```python
from build123d import *

# Parameters (mm, degrees)
F2_R      = 2
F3_DEPTH  = 20
F4_R      = 4
F5_DEPTH  = 20
F8_DEPTH  = 1.4
F9_R      = 3
F10_DEPTH = 8
F9_R_2    = 5
F11_DEPTH = 0.4


with BuildPart() as f1:
    # F0 (on Front) → F1 (revolve)
    with BuildSketch(Plane.XZ):
        Polygon((0, 15), (0, 0), (48, 0), (48, 4.5), (36, 4.5), (36, 7), (3, 7), (3, 11), (2.8, 11), (2.8, 15), align=None)
    revolve(axis=Axis((24, 0, 0), (-1, 0, 0)))

    # F2 (on face) → F3 (cut)
    with BuildSketch(Plane.YZ.offset(48)):
        Circle(F2_R)
    extrude(amount=-F3_DEPTH, mode=Mode.SUBTRACT)

    # F4 (on face) → F5 (cut)
    with BuildSketch(Plane(origin=(0, 0, 0), x_dir=(0, -1, 0), z_dir=(-1, 0, 0))):
        Circle(F4_R)
    extrude(amount=-F5_DEPTH, mode=Mode.SUBTRACT)

    # F7 (on offset) → F8 (cut)
    with BuildSketch(Plane.XY.offset(4.5)):
        with BuildLine():
            ThreePointArc((39, 1.5), (37.5, 0), (39, -1.5))
            Line((39, -1.5), (45, -1.5))
            ThreePointArc((45, -1.5), (46.5, 0), (45, 1.5))
            Line((45, 1.5), (39, 1.5))
        make_face()
    extrude(amount=-F8_DEPTH, mode=Mode.SUBTRACT)

    # F9 (on face) → F10 (join)
    with BuildSketch(Plane(origin=(0, 0, 0), x_dir=(0, -1, 0), z_dir=(-1, 0, 0))):
        with Locations((-9, 0)):
            Circle(F9_R)
    extrude(amount=F10_DEPTH)

    # F9 (on face) → F11 (join)
    with BuildSketch(Plane(origin=(0, 0, 0), x_dir=(0, -1, 0), z_dir=(-1, 0, 0))):
        with Locations((-9, 0)):
            Circle(F9_R_2)
        with Locations((-9, 0)):
            Circle(F9_R, mode=Mode.SUBTRACT)
    extrude(amount=F11_DEPTH)


solid = f1.part
```
Work out the finished part from the listing and answer in its coordinate system (mm). A direction names the side the tool comes from. Coordinates: 2 decimals unless noted, no trailing zeros. Loops run counter-clockwise (first coordinate to the right, second up) from the corner with the lowest first, then second, coordinate; pieces in that order, holes last.
1) For a pull along X with two mould halves and no side action, classify faces 4 (the cylindrical face through (19.269, -2.681, 6.466)), 5 (the flat face through (3, 0.2, -7.2)), 6 (the flat face through (42, 0, 3.1)) as +X half, -X half, draft (parallel to the pull), parting line (faces both ways), or undercut.
Results:
face 4: draft
face 5: +X half
face 6: undercut
2) Section C-C (z = -10.25) is taken. Give the vertices of the cut face in (x, y).
Results:
outline: (0, -10.95) - (2.8, -10.95) - (2.8, -3.99) - (3, -3.99) - (3, 3.99) - (2.8, 3.99) - (2.8, 10.95) - (0, 10.95) - close
3) For faces 1 (the flat face through (36, -5, 0)), 2 (the cylindrical face through (-0.2, 4.23, 1.5)), 3 (the cylindrical face through (37.5, 0, 3.8)), determine the directions among +Z, -Z, +X, -X, +Y, -Y from which every point of the face is accessible in a straight line to the end or side of a thin tool.
Results:
face 1: +X
face 2: -X
face 3: +Z
4) Section A-A (x = 41.5) is taken. Give the vertices of the cut face in (y, z), plus the area to 3 significant figures.
Results:
outline: (-1.5, 3.1) - (-1.5, 4.24) arc R4.5 ccw (long way) to (1.5, 4.24) - (1.5, 3.1) - close; hole circle Ø4 at (0, 0)
area: 47.1 mm2
5) Section B-B (y = 0) is taken. Give the vertices of the cut face in (x, z), plus the area to 3 significant figures.
Results:
outline: (0, -15) - (2.8, -15) - (2.8, -11) - (3, -11) - (3, -7) - (36, -7) - (36, -4.5) - (48, -4.5) - (48, -2) - (28, -2) - (28, 2) - (48, 2) - (48, 4.5) - (46.5, 4.5) - (46.5, 3.1) - (37.5, 3.1) - (37.5, 4.5) - (36, 4.5) - (36, 7) - (3, 7) - (3, 11) - (2.8, 11) - (2.8, 15) - (0, 15) - (0, 4) - (20, 4) - (20, -4) - (0, -4) - close
area: 406 mm2
6) Section D-D (x = 15) is taken. Give the vertices of the cut face in (y, z), plus the area to 3 significant figures.
Results:
outline: circle Ø14 at (0, 0); hole circle Ø8 at (0, 0)
area: 104 mm2
7) Flat-ended cylindrical pins translate along their axes: pin 1 (1.3 mm diameter, centred on x = 43, z = 3.5, fed in from +Y); pin 2 (3 mm diameter, centred on y = -7, z = 4.5, fed in from +X); pin 3 (1 mm diameter, centred on x = -2, z = 10, fed in from -Y) (1 decimal); pin 4 (1.2 mm diameter, centred on y = 0.5, z = 0, fed in from +X). Find the tip coordinate at first contact, or state that the pin passes through.
Results:
pin 1: stops at y = 3.48
pin 2: stops at x = 36
pin 3: passes through
pin 4: stops at x = 28
8) Consider probe 1 along Y at (x, z) = (14, 0); probe 2 along X at (y, z) = (9, 9); probe 3 along X at (y, z) = (-4.25, 9.5). Determine where each line is inside the solid, lowest interval first.
Results:
probe 1: y = -7 to -4, 4 to 7
probe 2: x = 0 to 2.8
probe 3: x = 0 to 3
